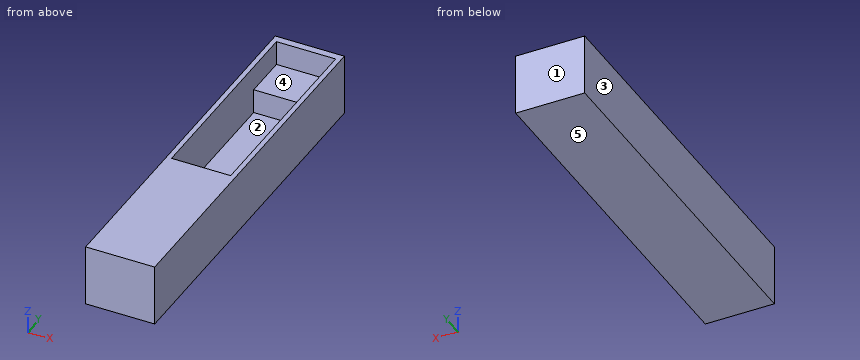
from build123d import *

# Parameters (mm, degrees)
F0_W     = 28
F0_H     = 25
F1_DEPTH = 150
F2_W     = 24
F2_H     = 18
F3_DEPTH = 10
F4_W     = 24
F4_H     = 65
F5_DEPTH = 20


with BuildPart() as f1:
    # F0 (on Front) → F1 (new body)
    with BuildSketch(Plane.XZ):
        with Locations((14, 12.5)):
            Rectangle(F0_W, F0_H)
    extrude(amount=F1_DEPTH)

    # F2 (on face) → F3 (cut)
    with BuildSketch(Plane.XY.offset(25)):
        with Locations((14, -12)):
            Rectangle(F2_W, F2_H)
    extrude(amount=-F3_DEPTH, mode=Mode.SUBTRACT)

    # F4 (on face) → F5 (cut)
    with BuildSketch(Plane.XY.offset(25)):
        with Locations((14, -53.5)):
            Rectangle(F4_W, F4_H)
    extrude(amount=-F5_DEPTH, mode=Mode.SUBTRACT)


solid = f1.part
Build history of the part. All positions in model axes, mm. Face numbers are marked on the shaded views. A direction names the side the tool comes from. Coordinates: 2 decimals unless noted, no trailing zeros. Order: outer loops, then holes, each group sorted by start corner. A loop starts at its lowest first (then second) coordinate and runs counter-clockwise, first axis right, second up. Notation, with made-up numbers: (42, 54) -> (84, 54) arc R5 cw to (84, 58) -> close; hole circle Ø7 at (0, 24.25). An arc over 180 degrees is marked (long way). One line per item, written item: value.
(1) Probe line 1 (X direction, y = -74, z = 8); line 2 (Y direction, x = 9.25, z = 22.5); line 3 (Y direction, x = 22.5, z = 11). List the from-to ranges inside material, lowest first. Write a range as [from, to].
Checked values:
line 1: [0, 2], [26, 28]
line 2: [-150, -86], [-3, 0]
line 3: [-150, -86], [-21, 0]
(2) Drop a flat-ended pin along its axis: pin 1 Ø9 at (x, y) = (16, -10) entering from +Z. Give the stop position or say it passes through.
Checked values:
pin 1: z = 15
(3) Tool access for the marked faces 4 and 5: list every direction of +Z, -Z, +X, -X, +Y, -Y with a clear straight run to the whole face (end or side of a thin tool).
Checked values:
face 4: +Z
face 5: -Z, +X, -X, +Y, -Y
(4) Slice it at D-D, the plane z = 20.5. List the corners of the cut face in (x, y), plus the area to 3 significant figures.
Checked values:
outline: (0, -150) -> (28, -150) -> (28, 0) -> (0, 0) -> close; hole (2, -86) -> (26, -86) -> (26, -3) -> (2, -3) -> close
area: 2,210 mm2
(5) Slice it at B-B, the plane x = 21. List the corners of the cut face in (y, z).
Checked values:
outline: (-150, 0) -> (0, 0) -> (0, 25) -> (-3, 25) -> (-3, 15) -> (-21, 15) -> (-21, 5) -> (-86, 5) -> (-86, 25) -> (-150, 25) -> close
(6) Slice it at A-A, the plane z = 13.75. List the corners of the cut face in (x, y), plus the area to 3 significant figures.
Checked values:
outline: (0, -150) -> (28, -150) -> (28, 0) -> (0, 0) -> close; hole (2, -86) -> (26, -86) -> (26, -21) -> (2, -21) -> close
area: 2,640 mm2
(7) Mould opens along X. For the marked faces 1, 2 and 3 say: pulls with the +X half, pulls with the -X half, needs draft (parallel to the pull), parting line crosses it, or undercut.
Checked values:
face 1: needs draft
face 2: undercut
face 3: pulls with the -X half
(8) Slice it at C-C, the plane y = -18.5. List the corners of the cut face in (x, z).
Checked values:
outline: (0, 0) -> (28, 0) -> (28, 25) -> (26, 25) -> (26, 15) -> (2, 15) -> (2, 25) -> (0, 25) -> close
